Input: dimensioned drawing with shaded views. Units: mm. Origin: part minimum x, y, z. A direction names the side the tool comes from. Round coordinates to 2 decimals unless told otherwise and drop trailing zeros. Loops run counter-clockwise (first coordinate to the right, second up) from the corner with the lowest first, then second, coordinate; pieces in that order, holes last. Notation, with made-up numbers: M 44,86.25 L 48,86.25 A19 ccw 48,120.25 Z; hole C -1,45 d10. An arc over 180 degrees is marked long. Return JSON: item names as keys, results as strings.
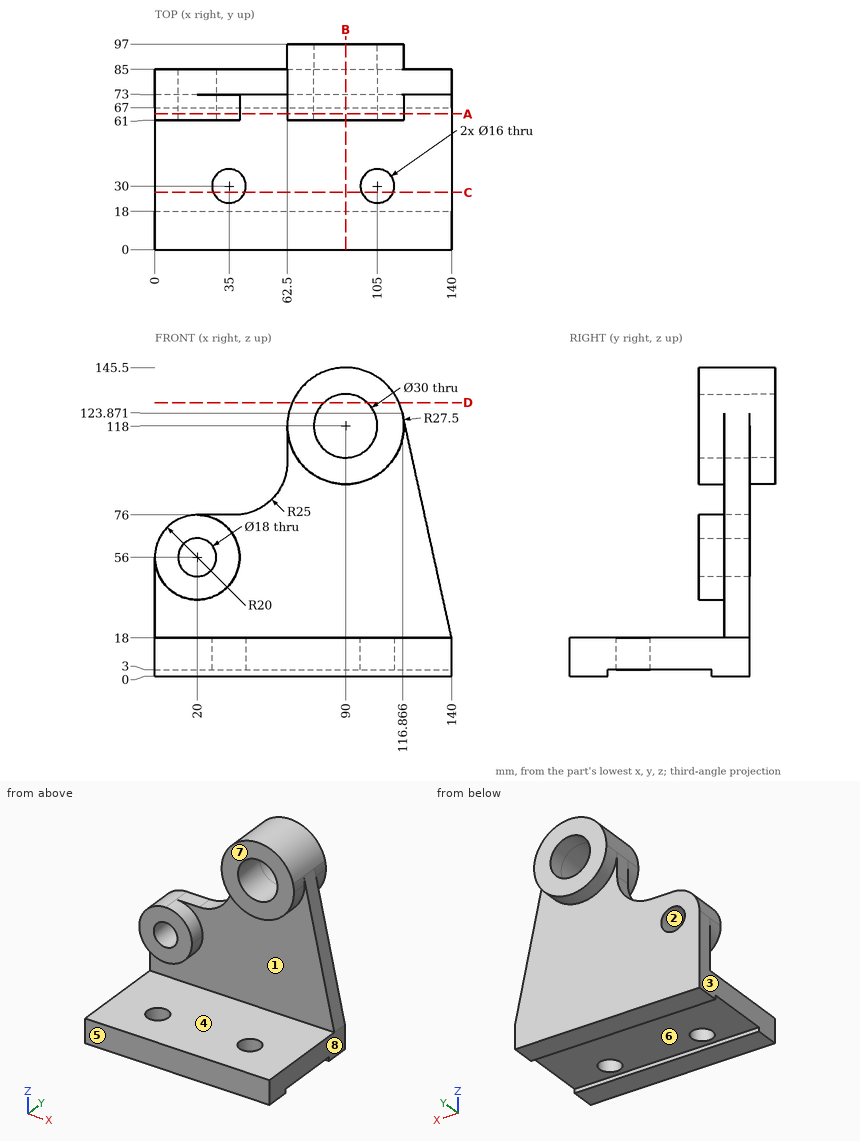
Q1. Section query A-A (y = 64). Output: boundary loops of the cut face in (x, z), plus the area to 3 significant figures.
Determined:
{"outline": "M 0,3 L 140,3 L 140,18 L 0,18 Z; M 0,56 A20 ccw 40,56 A20 ccw 20,76 A20 ccw Z; M 116.87,123.87 A27.5 ccw long 117.5,118 A27.5 ccw Z; hole C 20,56 d18; hole C 90,118 d30", "area": "4,770 mm^2"}
Q2. Section query D-D (z = 129). Output: boundary loops of the cut face in (x, y) (1 decimal), plus the area to 3 significant figures.
Determined:
{"outline": "M 64.8,61 L 79.8,61 L 79.8,97 L 64.8,97 Z; M 100.2,61 L 115.2,61 L 115.2,97 L 100.2,97 Z", "area": "1,080 mm^2"}
Q3. Pull-direction query (X, two-part tool) for the marked faces 1, 2 and 3; classes: pulls with the +X half, pulls with the -X half, needs draft (parallel to the pull), parting line crosses it, or undercut.
Determined:
{"face 1": "needs draft", "face 2": "undercut", "face 3": "pulls with the -X half"}
Q4. Reachability of the marked faces 4, 5, 6, 7 and 8 from +Z, -Z, +X, -X, +Y, -Y: full face, straight path, thin tool, end or side. Return the list, or none.
Determined:
{"face 4": "+X, -X, -Y", "face 5": "+Z, -Z, +X, -X, -Y", "face 6": "-Z, +X, -X", "face 7": "+Z, +X, -X, -Y", "face 8": "+Z, -Z, +X, +Y, -Y"}
Q5. Section query B-B (x = 90). Output: boundary loops of the cut face in (y, z), plus the area to 3 significant figures.
Determined:
{"outline": "M 0,0 L 18,0 L 18,3 L 67,3 L 67,0 L 85,0 L 85,90.5 L 97,90.5 L 97,103 L 61,103 L 61,90.5 L 73,90.5 L 73,18 L 0,18 Z; M 61,133 L 97,133 L 97,145.5 L 61,145.5 Z", "area": "3,150 mm^2"}
Q6. Section query C-C (y = 27). Output: boundary loops of the cut face in (x, z), plus the area to 4 significant figures.
Determined:
{"outline": "M 0,3 L 27.58,3 L 27.58,18 L 0,18 Z; M 42.42,3 L 97.58,3 L 97.58,18 L 42.42,18 Z; M 112.42,3 L 140,3 L 140,18 L 112.42,18 Z", "area": "1,655 mm^2"}
Q7. Pin query (flat end, axial travel): pin 1 (5 mm diameter, centred on x = 101.5, z = 17.5, fed in from +Y); pin 2 (5 mm diameter, centred on x = 41, y = 46.5, fed in from -Z); pin 3 (1 mm diameter, centred on x = 51, y = 47, fed in from +Z). Return the tip coordinate at first contact, or that it passes through.
Determined:
{"pin 1": "stops at y = 85", "pin 2": "stops at z = 3", "pin 3": "stops at z = 18"}
Q8. Material intervals for L1, parallel to Z at x = 90.5, y = 70.5 (1 decimal); L2, parallel to Z at x = 90, y = 90.25; L3, parallel to Z at x = 7.5, y = 32.5, sorted ascending.
Determined:
{"L1": "z = 0 to 18, 90.5 to 103, 133 to 145.5", "L2": "z = 90.5 to 103, 133 to 145.5", "L3": "z = 3 to 18"}
